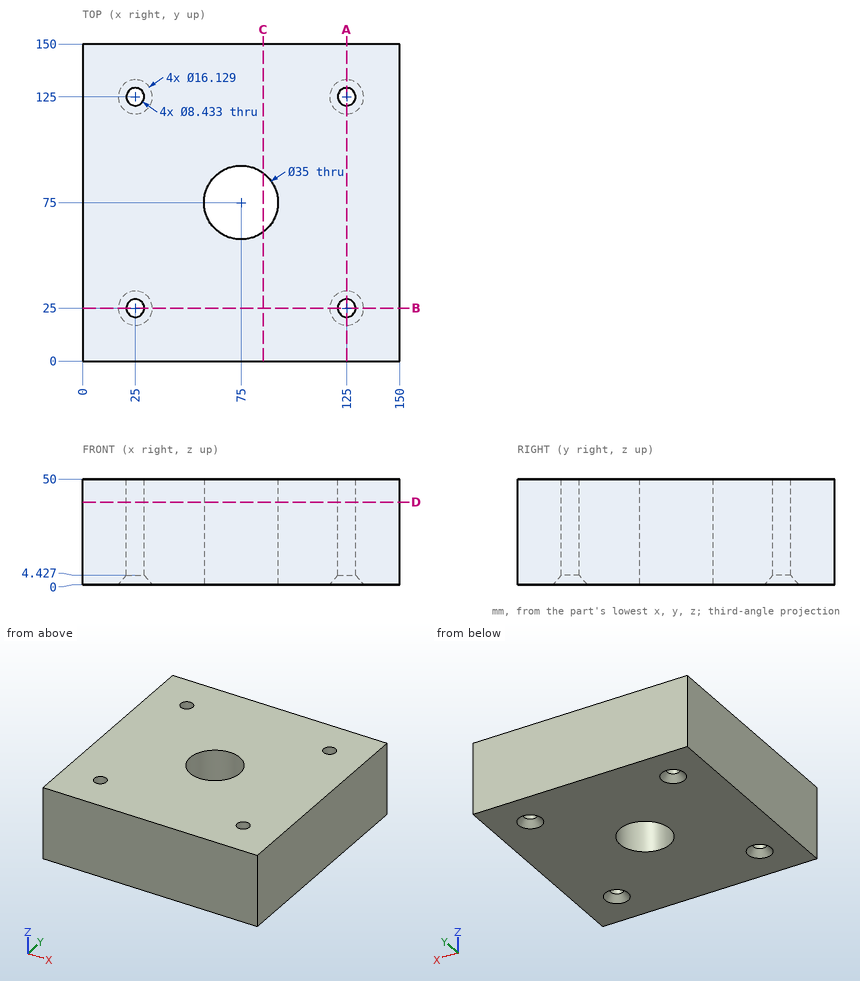
Study the drawing (mm; zero at the part's minimum x, y, z) and answer. Round coordinates to 2 decimals unless told otherwise and drop trailing zeros. Write each loop counter-clockwise with the first axis right and the second up, starting at its lowest first coordinate (ties: lowest second). Pieces come first, ordered by that corner, then holes. Notation, with made-up numbers: (75, -3) - (88, -3) arc R28 cw to (88, 31) - close; hole circle Ø4 at (50, 50.25). An arc over 180 degrees is marked (long way). Use a Markdown table: item, result. Add a question column.
1. The part is cut by section C-C (x = 85.5). Write down the section's boundary in (y, z), and give its area (3 significant figures).
2. The part is cut by section D-D (z = 39). Write down the section's boundary in (x, y), and give its area (3 significant figures).
3. Consider line 1 (Y direction, x = 25, z = 19); line 2 (X direction, y = 75, z = 23). Determine where each line is inside the solid, lowest interval first.
4. Flat-ended cylindrical pins translate along their axes: P1, Ø5, axis at x = 102, z = 11.5, coming from the -Y side; P2, Ø7.5, axis at x = 125, y = 25, coming from the -Z side; P3, Ø9.5, axis at x = 25, y = 25, coming from the -Z side. Find the tip coordinate at first contact, or state that the pin passes through.
5. The part is cut by section A-A (x = 125). Write down the section's boundary in (y, z) (1 decimal), and give its area (3 significant figures).
Reported:
| question | item | result |
|---|---|---|
| 1 | outline | (0, 0) - (61, 0) - (61, 50) - (0, 50) - close; (89, 0) - (150, 0) - (150, 50) - (89, 50) - close |
| 1 | area | 6,100 mm^2 |
| 2 | outline | (0, 0) - (150, 0) - (150, 150) - (0, 150) - close; hole circle Ø8.43 at (25, 25); hole circle Ø8.43 at (25, 125); hole circle Ø35 at (75, 75); hole circle Ø8.43 at (125, 25); hole circle Ø8.43 at (125, 125) |
| 2 | area | 21,300 mm^2 |
| 3 | line 1 | 0 to 20.78, 29.22 to 120.78, 129.22 to 150 |
| 3 | line 2 | 0 to 57.5, 92.5 to 150 |
| 4 | P1 | y = 0 |
| 4 | P2 | through |
| 4 | P3 | z = 3.81 |
| 5 | outline | (0, 0) - (16.9, 0) - (20.8, 4.4) - (20.8, 50) - (0, 50) - close; (29.2, 4.4) - (33.1, 0) - (116.9, 0) - (120.8, 4.4) - (120.8, 50) - (29.2, 50) - close; (129.2, 4.4) - (133.1, 0) - (150, 0) - (150, 50) - (129.2, 50) - close |
| 5 | area | 6,620 mm^2 |
